The drawing under review shows one solid part. Ordinate dimensions are in mm from its lowest x, y, z. A direction names the side the tool comes from. Give positions to 0.01 mm unless a question says otherwise; leave off trailing zeros. Write each loop counter-clockwise with the first axis right and the second up, starting at its lowest first coordinate (ties: lowest second). Pieces come first, ordered by that corner, then holes. Notation, with made-up numbers: (65, 66) -> (78, 66) arc R27 cw to (78, 100) -> close; hole circle Ø3 at (57.5, 79.25). An arc over 180 degrees is marked (long way). Put each result on its own line as item: value. Start each with the question number.
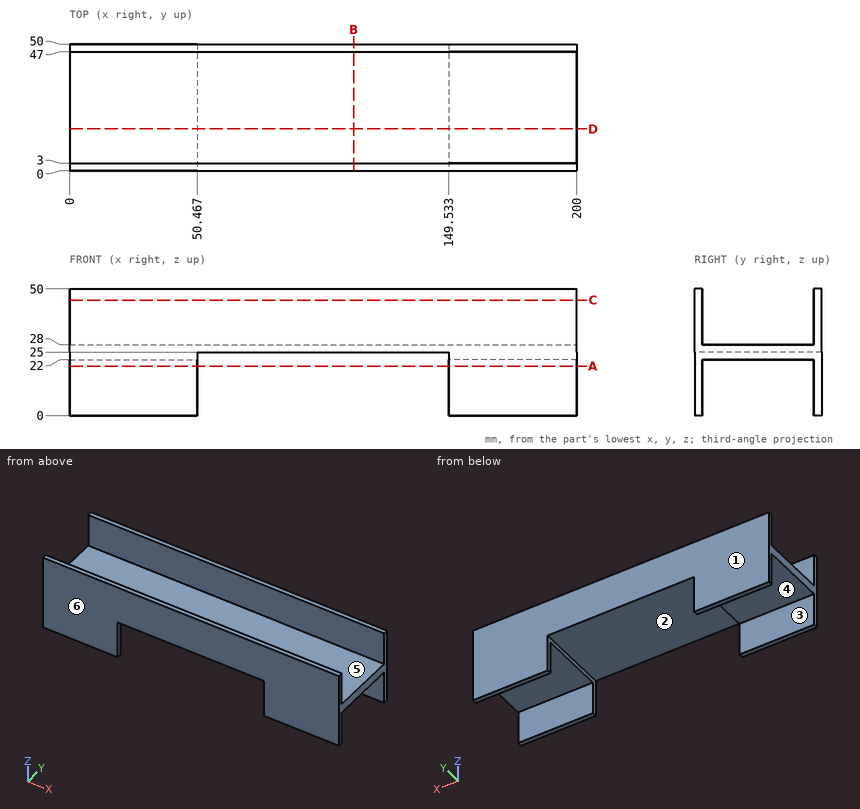
Q1. For pin 1 (7.5 mm diameter, centred on y = 26, z = 16, fed in from +X); pin 2 (3 mm diameter, centred on x = 53, y = 37.5, fed in from +Z); pin 3 (5 mm diameter, centred on x = 89, y = 18.5, fed in from -Z); pin 4 (13 mm diameter, centred on x = 178.5, y = 20, fed in from -Z), all flat-tipped, find the tip position at first contact; note any pin that passes through.
Q2. Mouldability with a two-part tool opening along Y and no side actions: class the marked faces 1, 2 and 3 as +Y half, -Y half, draft (parallel to the pull), parting line (faces both ways), or undercut.
Q3. Take a section at D-D on y = 16.5. Give the boundary of the cut face in (x, z).
Q4. To check wall thickness, follow probe 1 along Y at (x, z) = (49, 19.5); probe 2 along Z at (x, y) = (130.5, 40); probe 3 along Z at (x, y) = (164, 4.5). State the ranges of each line that lie inside material, in increasing order. Write a range as from..to.
Q5. Take a section at B-B on x = 112. Give the boundary of the cut face in (y, z), then the cut area to 3 significant figures.
Q6. Take a section at A-A on z = 19.5. Give the boundary of the cut face in (x, y).
Q7. Machinability: for the marked faces 4, 5 and 6, which of the approach directions +Z, -Z, +X, -X, +Y, -Y give a long, thin tool a straight path to every point of the face, cutting with its end or side? Answer none if there is none.
Q8. Take a section at C-C on z = 45.5. Give the boundary of the cut face in (x, y).
Result:
1. pin 1: passes through
1. pin 2: stops at z = 28
1. pin 3: stops at z = 25
1. pin 4: stops at z = 22
2. face 1: +Y half
2. face 2: draft
2. face 3: undercut
3. outline: (0, 22) -> (50.47, 22) -> (50.47, 25) -> (149.53, 25) -> (149.53, 22) -> (200, 22) -> (200, 28) -> (0, 28) -> close
4. probe 1: y = 0..3, 47..50
4. probe 2: z = 25..28
4. probe 3: z = 22..28
5. outline: (0, 25) -> (50, 25) -> (50, 50) -> (47, 50) -> (47, 28) -> (3, 28) -> (3, 50) -> (0, 50) -> close
5. area: 282 mm^2
6. outline: (0, 0) -> (50.47, 0) -> (50.47, 3) -> (0, 3) -> close; (0, 47) -> (50.47, 47) -> (50.47, 50) -> (0, 50) -> close; (149.53, 0) -> (200, 0) -> (200, 3) -> (149.53, 3) -> close; (149.53, 47) -> (200, 47) -> (200, 50) -> (149.53, 50) -> close
7. face 4: -Z, +X, -X
7. face 5: +Z, +X, -X
7. face 6: +Z, -Z, +X, -X, -Y
8. outline: (0, 0) -> (200, 0) -> (200, 3) -> (0, 3) -> close; (0, 47) -> (200, 47) -> (200, 50) -> (0, 50) -> close
